Here's how the part is built. I have some questions about the finished solid (model axes, mm). Face numbers are marked on the shaded views. A direction names the side the tool comes from. Coordinates: 2 decimals unless noted, no trailing zeros. Loops run counter-clockwise (first coordinate to the right, second up) from the corner with the lowest first, then second, coordinate; pieces in that order, holes last.
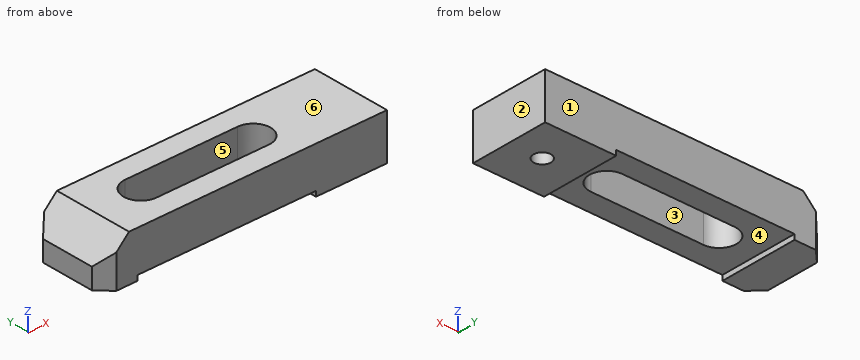
```python
from build123d import *

# Parameters (mm, degrees)
F0_W     = 111
F0_H     = 31
F1_DEPTH = 18
F3_DEPTH = 20
F4_R     = 3.4
F5_DEPTH = 12
F6_W     = 69.834876
F6_H     = 31
F7_DEPTH = 2
F8_SIZE  = 10
F9_SIZE  = 5


with BuildPart() as f1:
    # F0 (on Top) → F1 (new body)
    with BuildSketch(Plane.XY):
        Rectangle(F0_W, F0_H)
    extrude(amount=F1_DEPTH)

    # F2 (on face) → F3 (cut)
    with BuildSketch(Plane.XY.offset(18)):
        with BuildLine():
            Line((17.25, 6.75), (-26.75, 6.75))
            ThreePointArc((-26.75, 6.75), (-33.5, 0), (-26.75, -6.75))
            Line((-26.75, -6.75), (17.25, -6.75))
            ThreePointArc((17.25, -6.75), (24, 0), (17.25, 6.75))
        make_face()
    extrude(amount=-F3_DEPTH, mode=Mode.SUBTRACT)

    # F4 (on face) → F5 (cut)
    with BuildSketch(Plane(origin=(0, 0, 0), x_dir=(1, 0, 0), z_dir=(0, 0, -1))):
        with Locations((42.5, 0)):
            Circle(F4_R)
    extrude(amount=-F5_DEPTH, mode=Mode.SUBTRACT)

    # F6 (on face) → F7 (cut)
    with BuildSketch(Plane(origin=(0, 0, 0), x_dir=(1, 0, 0), z_dir=(0, 0, -1))):
        with Locations((-7.229885, 0)):
            Rectangle(F6_W, F6_H)
    extrude(amount=-F7_DEPTH, mode=Mode.SUBTRACT)

    # F8
    f8_edges = [f1.edges().sort_by_distance(p)[0] for p in [
        (-55.5, 0, 18),
    ]]
    chamfer(f8_edges, length=F8_SIZE)

    # F9
    f9_edges = [f1.edges().sort_by_distance(p)[0] for p in [
        (-55.5, -15.5, 4),
        (-55.5, 15.5, 4),
    ]]
    chamfer(f9_edges, length=F9_SIZE)


solid = f1.part
```
1. I need wall thicknesses on line 1 along X through (y, z) = (0, 5.5); line 2 along Y through (x, z) = (42.5, 8); line 3 along Y through (x, z) = (-13.5, 6.25). Which ranges of each line are inside material? Lowest first, please.
2. For pin 1 (1 mm diameter, centred on x = 23.5, y = -9.5, fed in from -Z); pin 2 (6 mm diameter, centred on x = 42.5, y = 0, fed in from -Z); pin 3 (6 mm diameter, centred on x = -20, y = -2.5, fed in from +Z), each with a flat end and sliding along its axis, tell me the tip position at first contact or that it passes through.
3. I want a section at B-B (x = 12.5). Please give me the cut outline in (y, z).
4. On a 3-axis mill with a long thin cutter (end or side, diameter ignored), from which of +Z, -Z, +X, -X, +Y, -Y can I reach the whole of each face in a straight line? I mean the marked faces 4, 5 and 6. Say none if no direction works.
5. We'd pull the mould along X, two halves only. Please class the marked faces 1, 2 and 3: +X half, -X half, draft (parallel to the pull), parting line (faces both ways), or undercut.
6. I want a section at C-C (y = 0). Please give me the cut outline in (x, z), then the cut area to 3 significant figures.
7. I want a section at A-A (z = 9.5). Please give me the cut outline in (x, y).
8. I want a section at D-D (x = 42.5). Please give me the cut outline in (y, z).
Response values:
1. line 1: x = -55.5 to -33.5, 24 to 39.1, 45.9 to 55.5
1. line 2: y = -15.5 to -3.4, 3.4 to 15.5
1. line 3: y = -15.5 to -6.75, 6.75 to 15.5
2. pin 1: stops at z = 2
2. pin 2: stops at z = 12
2. pin 3: passes through
3. outline: (-15.5, 2) - (-6.75, 2) - (-6.75, 18) - (-15.5, 18) - close; (6.75, 2) - (15.5, 2) - (15.5, 18) - (6.75, 18) - close
4. face 4: -Z, +Y, -Y
4. face 5: +Z, -Z
4. face 6: +Z, +X, -X, +Y, -Y
5. face 1: draft
5. face 2: +X half
5. face 3: undercut
6. outline: (-55.5, 0) - (-42.15, 0) - (-42.15, 2) - (-33.5, 2) - (-33.5, 18) - (-45.5, 18) - (-55.5, 8) - close; (24, 2) - (27.69, 2) - (27.69, 0) - (39.1, 0) - (39.1, 12) - (45.9, 12) - (45.9, 0) - (55.5, 0) - (55.5, 18) - (24, 18) - close
6. area: 807 mm2
7. outline: (-54, -12) - (-50.5, -15.5) - (55.5, -15.5) - (55.5, 15.5) - (-50.5, 15.5) - (-54, 12) - close; hole (-26.75, -6.75) - (17.25, -6.75) arc R6.75 ccw to (17.25, 6.75) - (-26.75, 6.75) arc R6.75 ccw to start; hole circle Ø6.8 at (42.5, 0)
8. outline: (-15.5, 0) - (-3.4, 0) - (-3.4, 12) - (3.4, 12) - (3.4, 0) - (15.5, 0) - (15.5, 18) - (-15.5, 18) - close
